from build123d import *

# Parameters (mm, degrees)
SKETCH1_R           = 0.889
SKETCH1_R_2         = 1.875
BOSS_EXTRUDE1_DEPTH = 8
SKETCH2_R           = 4
CUT_EXTRUDE1_DEPTH  = 5.5
FILLET1_R           = 1.5


with BuildPart() as part:
    # Sketch1 → Boss-Extrude1 (new body)
    with BuildSketch(Plane(origin=(0, 0, 0), x_dir=(1, 0, 0), z_dir=(0, 1, 0))):
        with BuildLine():
            Line((-7.071067812, 2.5), (-22, 2.5))
            Line((-22, 2.5), (-22, -2.5))
            Line((-22, -2.5), (-7.071067812, -2.5))
            ThreePointArc((-7.071067812, -2.5), (0, -7.5), (7.071067812, -2.5))
            Line((7.071067812, -2.5), (22, -2.5))
            Line((22, -2.5), (22, 2.5))
            Line((22, 2.5), (7.071067812, 2.5))
            ThreePointArc((7.071067812, 2.5), (0, 7.5), (-7.071067812, 2.5))
        make_face()
        with Locations(Location((-19.5, 0, 0), (0, 0, 270))):
            Circle(SKETCH1_R, mode=Mode.SUBTRACT)
        with Locations(Location((0, 0, 0), (0, 0, 270))):
            Circle(SKETCH1_R_2, mode=Mode.SUBTRACT)
        with Locations(Location((19.5, 0, 0), (0, 0, 270))):
            Circle(SKETCH1_R, mode=Mode.SUBTRACT)
        with Locations(Location((-14.5, 0, 0), (0, 0, 270))):
            Circle(SKETCH1_R, mode=Mode.SUBTRACT)
        with Locations(Location((14.5, 0, 0), (0, 0, 270))):
            Circle(SKETCH1_R, mode=Mode.SUBTRACT)
    extrude(amount=BOSS_EXTRUDE1_DEPTH)

    # Sketch2 → Cut-Extrude1 (cut)
    with BuildSketch(Plane(origin=(0, 8, 0), x_dir=(1, 0, 0), z_dir=(0, 1, 0))):
        with Locations(Location((0, 0, 0), (0, 0, 270))):
            Circle(SKETCH2_R)
    extrude(amount=-CUT_EXTRUDE1_DEPTH, mode=Mode.SUBTRACT)

    # Fillet1
    fillet1_edges = [part.edges().sort_by_distance(p)[0] for p in [
        (-19.5, 8, -0.889),
        (19.5, 8, -0.889),
    ]]
    fillet(fillet1_edges, radius=FILLET1_R)


solid = part.part
For this review, take the finished solid that the model builds, in its own axes (mm). A direction names the side the tool comes from. Coordinates: 2 decimals unless noted, no trailing zeros. Loops run counter-clockwise (first coordinate to the right, second up) from the corner with the lowest first, then second, coordinate; pieces in that order, holes last. Notation, with made-up numbers: (-23, 22) -> (-5, 22) arc R19 cw to (-5, 30) -> close; hole circle Ø1 at (51.5, 18). An arc over 180 degrees is marked (long way). Write each question's results on one line, items separated by ' | '.
Q1. Add section C-C, the plane z = 0. Count the separate pieces of the cut face and the enclosed holes in it, then the cut area to 3 significant figures.
Taken from the geometry:
separate pieces: 6 | enclosed holes: 0 | area: 240 mm²
Q2. To check wall thickness, follow line 1 along X through (y, z) = (1.1, 0) (3 decimals); line 2 along X through (y, z) = (4.5, 0); line 3 along Z through (x, y) = (0, 1.5) (3 decimals). State the ranges of each line that lie inside material, in increasing order. Write a range as [from, to].
Taken from the geometry:
line 1: [-22, -20.389], [-18.611, -15.389], [-13.611, -1.875], [1.875, 13.611], [15.389, 18.611], [20.389, 22] | line 2: [-22, -20.39], [-18.61, -15.39], [-13.61, -4], [4, 13.61], [15.39, 18.61], [20.39, 22] | line 3: [-7.5, -1.875], [1.875, 7.5]
Q3. Add section A-A, the plane y = 1. State the section outline as (x, z) points (3 decimals), then the cut area to 3 significant figures.
Taken from the geometry:
outline: (-22, -2.5) -> (-7.071, -2.5) arc R7.5 ccw to (7.071, -2.5) -> (22, -2.5) -> (22, 2.5) -> (7.071, 2.5) arc R7.5 ccw to (-7.071, 2.5) -> (-22, 2.5) -> close; hole circle Ø1.778 at (-19.5, 0); hole circle Ø1.778 at (-14.5, 0); hole circle Ø3.75 at (0, 0); hole circle Ø1.778 at (14.5, 0); hole circle Ø1.778 at (19.5, 0) | area: 302 mm²
Q4. For pin 1 Ø4 at (x, y) = (2.5, 1) entering from +Z; pin 2 Ø6.5 at (x, z) = (0, 0.5) entering from +Y; pin 3 Ø1 at (y, z) = (3, 6) entering from -X, all flat-tipped, find the tip position at first contact; note any pin that passes through.
Taken from the geometry:
pin 1: z = 7.48 | pin 2: y = 2.5 | pin 3: x = -5.1
Q5. Mouldability with a two-part tool opening along Z and no side actions: class faces 1 (the cylindrical face through (-18.62, 3.2, -0.12)), 2 (the flat face through (2, 8, -4)), 3 (the cylindrical face through (-0.1, 3.9, 7.5)) as +Z half, -Z half, draft (parallel to the pull), parting line (faces both ways), or undercut.
Taken from the geometry:
face 1: undercut | face 2: draft | face 3: +Z half
Q6. Machinability: for faces 4 (the flat face through (15, 4, -2.5)), 5 (the flat face through (14, 4, 2.5)), 6 (the cylindrical face through (-3.905, 5.288, -0.867)), 7 (the flat face through (-15, 4, 2.5)), which of the approach directions +Z, -Z, +X, -X, +Y, -Y give a long, thin tool a straight path to every point of the face, cutting with its end or side? Answer none if there is none.
Taken from the geometry:
face 4: -Z, +X, +Y, -Y | face 5: +Z, +X, +Y, -Y | face 6: +Y | face 7: +Z, -X, +Y, -Y
Q7. Add section B-B, the plane x = 14.5. State the section outline as (y, z) points.
Taken from the geometry:
outline: (0, -2.5) -> (8, -2.5) -> (8, -0.89) -> (0, -0.89) -> close; (0, 0.89) -> (8, 0.89) -> (8, 2.5) -> (0, 2.5) -> close
Q8. Add section D-D, the plane y = 5.5. State the section outline as (x, z) points.
Taken from the geometry:
outline: (-22, -2.5) -> (-7.07, -2.5) arc R7.5 ccw to (7.07, -2.5) -> (22, -2.5) -> (22, 2.5) -> (7.07, 2.5) arc R7.5 ccw to (-7.07, 2.5) -> (-22, 2.5) -> close; hole circle Ø1.78 at (-19.5, 0); hole circle Ø1.78 at (-14.5, 0); hole circle Ø8 at (0, 0); hole circle Ø1.78 at (14.5, 0); hole circle Ø1.78 at (19.5, 0)
